from build123d import *

# Parameters (mm, degrees)
SKETCH1_W           = 63.5
SKETCH1_H           = 57.15
SKETCH1_R           = 3.175
BOSS_EXTRUDE1_DEPTH = 5.08
SKETCH2_R           = 27.67
SKETCH2_R_2         = 24.13
BOSS_EXTRUDE2_DEPTH = 76.2
BOSS_EXTRUDE3_REACH = 59.15
SKETCH4_W           = 55.34
SKETCH4_H           = 50.8
SKETCH5_W           = 7.67
SKETCH5_H           = 3.2
BOSS_EXTRUDE4_DEPTH = 20
SKETCH6_R           = 2.5
CUT_EXTRUDE1_DEPTH  = 11
SKETCH7_W           = 7.67
SKETCH7_H           = 3.2
BOSS_EXTRUDE5_DEPTH = 2
SKETCH8_W           = 7.67
SKETCH8_H           = 2
BOSS_EXTRUDE6_DEPTH = 3.2


with BuildPart() as part:
    # Sketch1 → Boss-Extrude1 (new body)
    with BuildSketch(Plane(origin=(0, 0, 0), x_dir=(1, 0, 0), z_dir=(0, 1, 0))):
        with Locations((31.75, -28.575)):
            Rectangle(SKETCH1_W, SKETCH1_H)
        with Locations((6.35, -9.525)):
            Circle(SKETCH1_R, mode=Mode.SUBTRACT)
        with Locations((57.15, -9.525)):
            Circle(SKETCH1_R, mode=Mode.SUBTRACT)
        with Locations((57.15, -47.625)):
            Circle(SKETCH1_R, mode=Mode.SUBTRACT)
        with Locations((6.35, -47.625)):
            Circle(SKETCH1_R, mode=Mode.SUBTRACT)
    extrude(amount=BOSS_EXTRUDE1_DEPTH)

    # Sketch2 → Boss-Extrude2 (add)
    with BuildSketch(Plane(origin=(0, 5.08, 0), x_dir=(1, 0, 0), z_dir=(0, 1, 0))):
        with Locations((31.75, -28.575)):
            Circle(SKETCH2_R)
        with Locations((31.75, -28.575)):
            Circle(SKETCH2_R_2, mode=Mode.SUBTRACT)
    extrude(amount=BOSS_EXTRUDE2_DEPTH)

    # Sketch4 → Boss-Extrude3 (add, up to next)
    with BuildSketch(Plane(origin=(0, 0, 0), x_dir=(-1, 0, 0), z_dir=(0, 0, -1)), mode=Mode.PRIVATE) as boss_extrude3_sk1:
        with Locations((-31.75, 55.88)):
            Rectangle(SKETCH4_W, SKETCH4_H)
    boss_extrude3_tool1 = extrude(boss_extrude3_sk1.sketch, amount=-BOSS_EXTRUDE3_REACH, mode=Mode.PRIVATE) - part.part
    add(boss_extrude3_tool1.solids().sort_by_distance((31.75, 55.88, 0))[0])

    # Sketch5 → Boss-Extrude4 (add)
    with BuildSketch(Plane(origin=(0, 0, 0), x_dir=(-1, 0, 0), z_dir=(0, 0, -1))):
        with Locations((-7.915, 72.88)):
            Rectangle(SKETCH5_W, SKETCH5_H)
        with Locations((-55.585, 72.88)):
            Rectangle(SKETCH5_W, SKETCH5_H)
    extrude(amount=BOSS_EXTRUDE4_DEPTH)

    # Sketch6 → Cut-Extrude1 (cut, through all)
    with BuildSketch(Plane.XZ.offset(-71.28)):
        with Locations((7.45, -5.55)):
            Circle(SKETCH6_R)
        with Locations((56.05, -5.55)):
            Circle(SKETCH6_R)
        with Locations((56.05, -14.45)):
            Circle(SKETCH6_R)
        with Locations((7.45, -14.45)):
            Circle(SKETCH6_R)
    extrude(amount=-CUT_EXTRUDE1_DEPTH, mode=Mode.SUBTRACT)

    # Sketch7 → Boss-Extrude5 (add)
    with BuildSketch(Plane(origin=(0, 0, -20), x_dir=(-1, 0, 0), z_dir=(0, 0, -1))):
        with Locations((-55.585, 72.88)):
            Rectangle(SKETCH7_W, SKETCH7_H)
        with Locations((-7.915, 72.88)):
            Rectangle(SKETCH7_W, SKETCH7_H)
    extrude(amount=BOSS_EXTRUDE5_DEPTH)

    # Sketch8 → Boss-Extrude6 (add)
    with BuildSketch(Plane.XZ.offset(-71.28)):
        with Locations((7.915, -21)):
            Rectangle(SKETCH8_W, SKETCH8_H)
        with Locations((55.585, -21)):
            Rectangle(SKETCH8_W, SKETCH8_H)
    extrude(amount=BOSS_EXTRUDE6_DEPTH)


solid = part.part
Source: CAD feature listing. Evaluate the final solid. Frame: model axes, mm. A direction names the side the tool comes from. Round coordinates to 2 decimals unless told otherwise and drop trailing zeros. Loops run counter-clockwise (first coordinate to the right, second up) from the corner with the lowest first, then second, coordinate; pieces in that order, holes last.
Q1. Access query for faces 1 (the face through (8, 70, -20)), 2 (the face through (53.978, 2.504, 9.385)), 3 (the face through (8, 68.08, -21)). Directions: +Z, -Z, +X, -X, +Y, -Y. A direction counts if a zero-diameter tool reaches every point of the face in a straight line with its end or side. Return the directions, or none.
Q2. Section B-B, the plane x = 57.15. State how many separate pieces and enclosed holes the cut face has, plus the area to 3 significant figures.
Q3. Section C-C, the plane y = 51. Return loops of the section in (x, z) (3 decimals), plus the area to 3 significant figures.
Q4. First-contact query: P1, Ø1.6, axis at x = 8.5, y = 70, coming from the +Z side; P2, Ø12, axis at y = 10.5, z = 6, coming from the -X side; P3, Ø1, axis at x = 9, z = -21, coming from the -Y side; P4, Ø10, axis at x = 8.5, y = 63.5, coming from the +Z side. Flat tips, straight axial feed; report the tip coordinate or a pass-through.
Q5. Mould query, pull axis Y, two halves, no side actions, for faces 4 (the face through (58.36, 72.86, -15.41)), 5 (the face through (27, 5.08, 56)), 6 (the face through (56, 68.08, -21)), 7 (the face through (32, 81.28, 3)). Classes: pulls with the +Y half, pulls with the -Y half, needs draft (parallel to the pull), parting line crosses it, or undercut.
Q6. Section D-D, the plane x = 31.75. Return loops of the section in (y, z) (3 decimals), plus the area to 3 significant figures.
Q7. Ray query, line 1 (Z direction, x = 6.35, y = 3.4); line 2 (Y direction, x = 21.5, z = 1); line 3 (X direction, y = 23, z = 27.5). Return the intervals inside material, ascending.
Q8. Section A-A, the plane z = -5.55. Return loops of the section in (x, y), plus the area to 3 significant figures.
Solutions:
1. face 1: +X, -X, -Y
1. face 2: -Y
1. face 3: -Z, +X, -X, -Y
2. separate pieces: 5
2. enclosed holes: 0
2. area: 2,840 mm2
3. outline: (4.08, 0) - (59.42, 0) - (59.42, 28.575) arc R27.67 ccw to (4.08, 28.575) - close; hole circle Ø48.26 at (31.75, 28.575)
3. area: 955 mm2
4. P1: stops at z = 44.75
4. P2: stops at x = 0
4. P3: stops at y = 68.08
4. P4: stops at z = 49.37
5. face 4: needs draft
5. face 5: undercut
5. face 6: pulls with the -Y half
5. face 7: pulls with the +Y half
6. outline: (0, 0) - (5.08, 0) - (5.08, 0.905) - (30.48, 0.905) - (30.48, 0) - (81.28, 0) - (81.28, 4.445) - (5.08, 4.445) - (5.08, 52.705) - (81.28, 52.705) - (81.28, 56.245) - (5.08, 56.245) - (5.08, 57.15) - (0, 57.15) - close
6. area: 876 mm2
7. line 1: z = 0 to 6.35, 12.7 to 44.45, 50.8 to 57.15
7. line 2: y = 0 to 5.08, 30.48 to 81.28
7. line 3: x = 4.1 to 7.64, 55.86 to 59.4
8. outline: (4.08, 71.28) - (4.95, 71.28) - (4.95, 74.48) - (4.08, 74.48) - close; (9.95, 71.28) - (11.75, 71.28) - (11.75, 74.48) - (9.95, 74.48) - close; (51.75, 71.28) - (53.55, 71.28) - (53.55, 74.48) - (51.75, 74.48) - close; (58.55, 71.28) - (59.42, 71.28) - (59.42, 74.48) - (58.55, 74.48) - close
8. area: 17.1 mm2
